Here's how the part is built. I have some questions about the finished solid (model axes, mm). Coordinates: 2 decimals unless noted, no trailing zeros. Write each loop counter-clockwise with the first axis right and the second up, starting at its lowest first coordinate (ties: lowest second). Pieces come first, ordered by that corner, then holes.
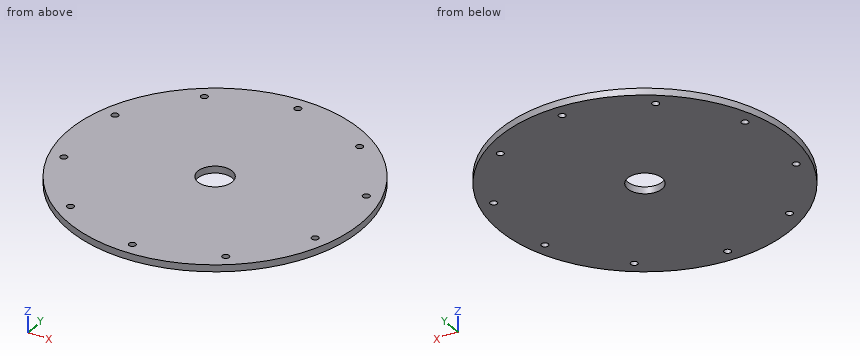
Solid Edge part; units mm, degrees
sketch "Sketch1" plane through (0, 0, 0) normal (0, 0, 1) x (1, 0, 0)
  circle A0 centre (-68.9258, 50.0648) radius 212.5
extrude "Protrusion1" add sketch "Sketch1" along normal blind 10
sketch "Sketch2" plane through (-68.9258, 50.0648, 10) normal (0, 0, 1) x (1, 0, 0)
  circle A0 centre (0, 192.5) radius 5
extrude "Cutout1" cut sketch "Sketch2" against normal through all
pattern_circular "Pattern1" count 10 over 360 about axis through (-68.9258, 50.0648, 10) along (0, 0, -1) of "Cutout1"
sketch "Sketch3" plane through (-68.9258, 50.0648, 10) normal (0, 0, 1) x (1, 0, 0)
  circle A0 centre (0, 0) radius 25
extrude "Cutout2" cut sketch "Sketch3" against normal through all
1) I need wall thicknesses on probe 1 along X at (y, z) = (209, 3.5); probe 2 along X at (y, z) = (-102, 6); probe 3 along X at (y, z) = (57.5, 2.75). Which ranges of each line are inside material? Lowest first, please.
Values follow:
probe 1: x = -209.98 to -185.92, -178.23 to 40.38, 48.07 to 72.13
probe 2: x = -217.36 to -185.47, -178.68 to 40.83, 47.62 to 79.51
probe 3: x = -281.3 to -92.79, -45.06 to 143.44
2) Imagine slicing it at A-A on z = 2.5. Count the separate pieces of the cut face and the enclosed holes in it, then the cut area to 3 significant figures.
Values follow:
separate pieces: 1
enclosed holes: 11
area: 139,000 mm2
3) Imagine slicing it at C-C on y = -68.5. Please give me the cut outline in (x, z).
Values follow:
outline: (-245.27, 0) - (107.42, 0) - (107.42, 10) - (-245.27, 10) - close
4) Will these pins go through, and if not, where does the flat tip stop? pin 1 (3 mm diameter, centred on x = -41.5, z = 7.5, fed in from +Y); pin 2 (1 mm diameter, centred on y = -100, z = 2.5, fed in from -X); pin 3 (6 mm diameter, centred on x = -145.5, z = 3.5, fed in from +Y).
Values follow:
pin 1: stops at y = 260.98
pin 2: stops at x = -219.88
pin 3: stops at y = 249.42
5) Imagine slicing it at B-B on x = 32.5. Please give me the cut outline in (y, z), then the cut area to 3 significant figures.
Values follow:
outline: (-136.67, 0) - (236.8, 0) - (236.8, 10) - (-136.67, 10) - close
area: 3,730 mm2
